Build history of the part. All positions in model axes, mm. A direction names the side the tool comes from. Give positions to 0.01 mm unless a question says otherwise; leave off trailing zeros. Write each loop counter-clockwise with the first axis right and the second up, starting at its lowest first coordinate (ties: lowest second). Pieces come first, ordered by that corner, then holes. Notation, with made-up numbers: (28.5, 17.5) -> (54.5, 17.5) arc R17 ccw to (54.5, 33.5) -> close; hole circle Ø8 at (24, 68.25). An arc over 180 degrees is marked (long way). Put each result on its own line as item: value. Start each with the question number.
Item 1: Slice it at A-A, the plane y = 15.24. List the corners of the cut face in (x, z) (3 decimals).
Item 2: Slice it at C-C, the plane z = 1.25. Give the number of separate pieces and of enclosed holes in the cut face, plus the area to 3 significant figures.
Item 3: Tool access for faces 1 (the flat face through (3, 8.89, 3)), 2 (the flat face through (57.15, 3, 3)), 3 (the flat face through (47.7, 11, 3)), 4 (the flat face through (82.55, 15, 3)): list every direction of +Z, -Z, +X, -X, +Y, -Y with a clear straight run to the whole face (end or side of a thin tool).
Item 4: Slice it at B-B, the plane y = 3.5. List the corners of the cut face in (x, z).
Item 5: Two-plate mould, pull along Y, no slides. Class faces 5 (the flat face through (47, 10.16, 3)), 6 (the flat face through (0, 26, 3)), 7 (the flat face through (73, 0, 3)): pulls with the +Y half, pulls with the -Y half, needs draft (parallel to the pull), parting line crosses it, or undercut.
Item 6: Slice it at D-D, the plane x = 55. List the corners of the cut face in (y, z).
Item 7: Drill centre lines: line 1 along Y through (x, z) = (66.5, 5.25); line 2 along Y through (x, z) = (84, 0.75); line 3 along X through (y, z) = (4, 2.5). Where is each one in solid material? Low to high.
Item 8: Flat gauge pins, fed straight in: pin 1 Ø4 at (x, y) = (70.5, 7.5) entering from -Z; pin 2 Ø1.9 at (x, z) = (52, 4) entering from -Y; pin 3 Ø1.5 at (y, z) = (20.5, 5) entering from -X; pin 4 Ø0.6 at (y, z) = (11, 2) entering from +X. Where does each tip first touch, or does it go through?
```python
from build123d import *

# Parameters (mm, degrees)
BOSS_EXTRUDE1_DEPTH = 6.35
SKETCH2_R           = 1.5
SKETCH2_W           = 25.4
SKETCH2_H           = 6.35
CUT_EXTRUDE1_DEPTH  = 7.35
CUT_EXTRUDE2_DEPTH  = 7.35


with BuildPart() as part:
    # Sketch1 → Boss-Extrude1 (new body)
    with BuildSketch(Plane.XY):
        Polygon((0, 21.59), (0, 30.48), (88.9, 30.48), (88.9, 21.59), (82.55, 21.59), (82.55, 8.89), (88.9, 8.89), (88.9, 0), (0, 0), (0, 8.89), (6.35, 8.89), (6.35, 21.59), align=None)
    extrude(amount=BOSS_EXTRUDE1_DEPTH)

    # Sketch2 → Cut-Extrude1 (cut, through all)
    with BuildSketch(Plane.XY.offset(6.35)):
        with Locations((22.225, 15.24)):
            Circle(SKETCH2_R)
        with Locations((66.675, 15.24)):
            Circle(SKETCH2_R)
        with Locations((44.45, 3.175)):
            Rectangle(SKETCH2_W, SKETCH2_H)
    extrude(amount=-CUT_EXTRUDE1_DEPTH, mode=Mode.SUBTRACT)

    # Sketch3 → Cut-Extrude2 (cut, through all)
    with BuildSketch(Plane.XY.offset(6.35)):
        Polygon((43.2, 6.35), (45.7, 6.35), (45.7, 10.16), (47.7, 10.16), (47.7, 12.16), (45.7, 12.16), (45.7, 16.51), (43.2, 16.51), (43.2, 12.16), (41.2, 12.16), (41.2, 10.16), (43.2, 10.16), align=None)
    extrude(amount=-CUT_EXTRUDE2_DEPTH, mode=Mode.SUBTRACT)


solid = part.part
```
Values follow:
1. outline: (6.35, 0) -> (20.725, 0) -> (20.725, 6.35) -> (6.35, 6.35) -> close; (23.725, 0) -> (43.2, 0) -> (43.2, 6.35) -> (23.725, 6.35) -> close; (45.7, 0) -> (65.175, 0) -> (65.175, 6.35) -> (45.7, 6.35) -> close; (68.175, 0) -> (82.55, 0) -> (82.55, 6.35) -> (68.175, 6.35) -> close
2. separate pieces: 1
2. enclosed holes: 2
2. area: 2,340 mm2
3. face 1: +Z, -Z, -X
3. face 2: +Z, -Z, -Y
3. face 3: +Z, -Z
3. face 4: +Z, -Z, +X
4. outline: (0, 0) -> (31.75, 0) -> (31.75, 6.35) -> (0, 6.35) -> close; (57.15, 0) -> (88.9, 0) -> (88.9, 6.35) -> (57.15, 6.35) -> close
5. face 5: undercut
5. face 6: needs draft
5. face 7: pulls with the -Y half
6. outline: (6.35, 0) -> (30.48, 0) -> (30.48, 6.35) -> (6.35, 6.35) -> close
7. line 1: 0 to 13.75, 16.73 to 30.48
7. line 2: 0 to 8.89, 21.59 to 30.48
7. line 3: 0 to 31.75, 57.15 to 88.9
8. pin 1: z = 0
8. pin 2: y = 6.35
8. pin 3: x = 6.35
8. pin 4: x = 82.55
